```python
from build123d import *

# Parameters (mm, degrees)
F0_W     = 50.8
F0_H     = 50.8
F1_DEPTH = 127
F2_R     = 6.35
F3_DEPTH = 177.8


with BuildPart() as f1:
    # F0 (on Top) → F1 (new body)
    with BuildSketch(Plane.XY):
        with Locations((25.4, -25.4)):
            Rectangle(F0_W, F0_H)
    extrude(amount=F1_DEPTH)

    # F2 (on face) → F3 (cut)
    with BuildSketch(Plane.XY.offset(127)):
        with Locations((25.4, -25.4)):
            Circle(F2_R)
        Polygon((19.84375, -47.625), (19.58975, -50.8), (31.21025, -50.8), (30.95625, -47.625), (34.13125, -47.625), (34.13125, -36.5125), (16.66875, -36.5125), (16.66875, -47.625), align=None)
        Polygon((50.8, -31.21025), (50.8, -19.58975), (47.625, -19.84375), (47.625, -16.66875), (36.5125, -16.66875), (36.5125, -34.13125), (47.625, -34.13125), (47.625, -30.95625), align=None)
        Polygon((3.175, -19.84375), (0, -19.58975), (0, -31.21025), (3.175, -30.95625), (3.175, -34.13125), (14.2875, -34.13125), (14.2875, -16.66875), (3.175, -16.66875), align=None)
        Polygon((19.84375, -3.175), (16.66875, -3.175), (16.66875, -14.2875), (34.13125, -14.2875), (34.13125, -3.175), (30.95625, -3.175), (31.21025, 0), (19.58975, 0), align=None)
    extrude(amount=-F3_DEPTH, mode=Mode.SUBTRACT)


solid = f1.part
```
Model file for the job. Use its own axes, mm. A direction names the side the tool comes from. Coordinates: 2 decimals unless noted, no trailing zeros. Write each loop counter-clockwise with the first axis right and the second up, starting at its lowest first coordinate (ties: lowest second). Pieces come first, ordered by that corner, then holes. Notation, with made-up numbers: (78, 0) - (108, 0) arc R22 ccw to (108, 28) - close; hole circle Ø9 at (-2.75, 48.25). An arc over 180 degrees is marked (long way). One line per question, with ' | ' between items. Start each with the question number.
Q1. Cut at B-B, the plane y = -46. List the corners of the cut face in (x, z).
Q2. 3-axis set-ups, long thin cutter, end or side, ignore diameter. For faces 1 (the face through (49.19, -31.08, 64.39)), 2 (the face through (18, -47.625, 64)), 3 (the face through (19.715, -1.565, 64.389)), 4 (the face through (1.565, -31.085, 64.389)): which of +Z, -Z, +X, -X, +Y, -Y reach the whole face in a straight line?
Q3. Cut at A-A, the plane x = 25.4. List the corners of the cut face in (y, z), then the cut area to 3 significant figures.
Q4. Pull direction Y, two halves, no side cores. Call faces 5 (the face through (47.625, -33, 64)), 6 (the face through (26, -36.512, 64)), 7 (the face through (50.8, -41, 63)), 8 (the face through (41, 0, 63)): pulls with the +Y half, pulls with the -Y half, needs draft (parallel to the pull), parting line crosses it, or undercut.
Q5. Drill centre lines: line 1 (X direction, y = -33.5, z = 68.5) (1 decimal); line 2 (Y direction, x = 33, z = 24) (1 decimal); line 3 (Y direction, x = 25, z = 52). Where is each one in solid material? Low to high. Write a range as [from, to].
Answer below:
1) outline: (0, 0) - (16.67, 0) - (16.67, 127) - (0, 127) - close; (34.13, 0) - (50.8, 0) - (50.8, 127) - (34.13, 127) - close
2) face 1: +Z, -Z, +X | face 2: +Z, -Z | face 3: +Z, -Z, +Y | face 4: +Z, -Z, -X
3) outline: (-36.51, 0) - (-31.75, 0) - (-31.75, 127) - (-36.51, 127) - close; (-19.05, 0) - (-14.29, 0) - (-14.29, 127) - (-19.05, 127) - close | area: 1,210 mm^2
4) face 5: undercut | face 6: undercut | face 7: needs draft | face 8: pulls with the +Y half
5) line 1: [0, 3.2], [14.3, 36.5], [47.6, 50.8] | line 2: [-50.8, -47.6], [-36.5, -14.3], [-3.2, 0] | line 3: [-36.51, -31.74], [-19.06, -14.29]
